from build123d import *

# Parameters (mm, degrees)
SKETCH1_W           = 260
SKETCH1_H           = 160
BOSS_EXTRUDE1_DEPTH = 10
SKETCH2_W           = 30
SKETCH2_H           = 10
BOSS_EXTRUDE2_DEPTH = 22
SKETCH3_R           = 1.5
CUT_EXTRUDE1_DEPTH  = 112
SKETCH4_W           = 30
SKETCH4_H           = 2.519449054
BOSS_EXTRUDE3_DEPTH = 10
SKETCH5_R           = 3.25
CUT_EXTRUDE4_DEPTH  = 10
SKETCH7_W           = 10
SKETCH7_H           = 10
CUT_EXTRUDE5_DEPTH  = 10
FILLET1_R           = 5
FILLET2_R           = 3


with BuildPart() as part:
    # Sketch1 → Boss-Extrude1 (new body)
    with BuildSketch(Plane(origin=(0, 0, 0), x_dir=(1, 0, 0), z_dir=(0, 1, 0))):
        Rectangle(SKETCH1_W, SKETCH1_H)
    extrude(amount=BOSS_EXTRUDE1_DEPTH)

    # Sketch2 → Boss-Extrude2 (add)
    with BuildSketch(Plane.XZ):
        with Locations((-65, 56)):
            Rectangle(SKETCH2_W, SKETCH2_H)
        with Locations((65, 56)):
            Rectangle(SKETCH2_W, SKETCH2_H)
        with Locations((65, -56)):
            Rectangle(SKETCH2_W, SKETCH2_H)
        with Locations((-65, -56)):
            Rectangle(SKETCH2_W, SKETCH2_H)
    extrude(amount=BOSS_EXTRUDE2_DEPTH)

    # Sketch3 → Cut-Extrude1 (cut)
    with BuildSketch(Plane.XY.offset(61)):
        with Locations((-65, -2.25)):
            Circle(SKETCH3_R)
        with Locations(Location((-65, -19.75, 0), (0, 0, 180))):
            Circle(SKETCH3_R)
        with Locations((65, -19.75)):
            Circle(SKETCH3_R)
        with Locations(Location((65, -2.25, 0), (0, 0, 180))):
            Circle(SKETCH3_R)
    cut_extrude1 = extrude(amount=-CUT_EXTRUDE1_DEPTH, mode=Mode.SUBTRACT)

    # Mirror1: Cut-Extrude1 across plane
    add(cut_extrude1.mirror(Plane.XY), mode=Mode.SUBTRACT)

    # Sketch4 → Boss-Extrude3 (add)
    with BuildSketch(Plane.XY.offset(61)):
        with Locations((-65, -23.259724527)):
            Rectangle(SKETCH4_W, SKETCH4_H)
        with Locations((65, -23.259724527)):
            Rectangle(SKETCH4_W, SKETCH4_H)
    boss_extrude3 = extrude(amount=-BOSS_EXTRUDE3_DEPTH)

    # Mirror3: Boss-Extrude3 across plane
    add(boss_extrude3.mirror(Plane.XY))

    # Sketch5 → Cut-Extrude4 (cut)
    with BuildSketch(Plane(origin=(0, 10, 0), x_dir=(1, 0, 0), z_dir=(0, 1, 0))):
        with Locations(Location((-36.593545043, 52.5, 0), (0, 0, 270))):
            Circle(SKETCH5_R)
        with Locations(Location((106.593545043, 52.5, 0), (0, 0, 270))):
            Circle(SKETCH5_R)
        with Locations(Location((-36.593545043, -52.5, 0), (0, 0, 270))):
            Circle(SKETCH5_R)
        with Locations(Location((106.593545043, -52.5, 0), (0, 0, 270))):
            Circle(SKETCH5_R)
    extrude(amount=-CUT_EXTRUDE4_DEPTH, mode=Mode.SUBTRACT)

    # Sketch7 → Cut-Extrude5 (cut)
    with BuildSketch(Plane(origin=(0, 10, 0), x_dir=(1, 0, 0), z_dir=(0, 1, 0))):
        with Locations((-5, 65)):
            Rectangle(SKETCH7_W, SKETCH7_H)
        with Locations((15, 65)):
            Rectangle(SKETCH7_W, SKETCH7_H)
    cut_extrude5 = extrude(amount=-CUT_EXTRUDE5_DEPTH, mode=Mode.SUBTRACT)

    # Mirror4: Cut-Extrude5 across plane
    add(cut_extrude5.mirror(Plane(origin=(0, 0, 0), x_dir=(1, 0, 0), z_dir=(0, 0, -1))), mode=Mode.SUBTRACT)

    # Fillet1
    fillet1_edges = [part.edges().sort_by_distance(p)[0] for p in [
        (130, 5, 80),
        (-130, 5, 80),
        (-130, 5, -80),
        (130, 5, -80),
    ]]
    fillet(fillet1_edges, radius=FILLET1_R)

    # Fillet2
    fillet2_edges = [part.edges().sort_by_distance(p)[0] for p in [
        (-10, 5, -60),
        (-10, 5, -70),
        (0, 5, -70),
        (0, 5, -60),
        (20, 5, -60),
        (10, 5, -60),
        (10, 5, -70),
        (20, 5, -70),
        (0, 5, 70),
        (0, 5, 60),
        (-10, 5, 60),
        (-10, 5, 70),
        (10, 5, 70),
        (20, 5, 70),
        (20, 5, 60),
        (10, 5, 60),
    ]]
    fillet(fillet2_edges, radius=FILLET2_R)


solid = part.part
Input: part model. Units: mm. Frame: model coordinates. A direction names the side the tool comes from. Give positions to 0.01 mm unless a question says otherwise; leave off trailing zeros. Order: outer loops, then holes, each group sorted by start corner. A loop starts at its lowest first (then second) coordinate and runs counter-clockwise, first axis right, second up. Notation, with made-up numbers: (-33.75, 58) - (-29.75, 58) arc R30 cw to (-29.75, 82) - close; hole circle Ø11 at (39, -33.75). An arc over 180 degrees is marked (long way). Write each question's results on one line, items separated by ' | '.
Item 1: Contact query for flat-ended pins moving along their axis: pin 1 Ø7.5 at (x, y) = (62.5, -9) entering from -Z; pin 2 Ø4 at (x, z) = (-96, 16.5) entering from -Y; pin 3 Ø7.5 at (x, y) = (63.5, -9) entering from +Z. Output: stop coordinate, or through.
A:
pin 1: stops at z = -61 | pin 2: stops at y = 0 | pin 3: stops at z = 61
Item 2: Draft query along Z for faces 5 (the cylindrical face through (105.349, 5.07, -49.498)), 6 (the cylindrical face through (-33.853, 5.07, -50.753)), 7 (the flat face through (-2, 5, 80)), 8 (the flat face through (-65, -24.519, -56)). Return one class per face: released by +Z, released by -Z, zero draft, split by the parting line, or undercut.
A:
face 5: undercut | face 6: undercut | face 7: released by +Z | face 8: zero draft
Item 3: Access query for faces 1 (the flat face through (65, -12, -51)), 2 (the flat face through (-65, -12, -61)), 3 (the flat face through (-80, -12, 56)), 4 (the flat face through (-50, -12, -56)). Directions: +Z, -Z, +X, -X, +Y, -Y. A direction counts if a zero-diameter tool reaches every point of the face in a straight line with its end or side. Return the directions, or none.
A:
face 1: +X, -X, -Y | face 2: -Z, +X, -X, -Y | face 3: +Z, -Z, -X, -Y | face 4: +Z, -Z, -Y
Item 4: Section C-C (x = 37). Return loops of the section in (y, z).
A:
outline: (0, -80) - (10, -80) - (10, 80) - (0, 80) - close
Item 5: Section A-A (y = -8.5). Return loops of the section in (x, z), and give its area (3 significant figures).
A:
outline: (-80, -61) - (-50, -61) - (-50, -51) - (-80, -51) - close; (-80, 51) - (-50, 51) - (-50, 61) - (-80, 61) - close; (50, -61) - (80, -61) - (80, -51) - (50, -51) - close; (50, 51) - (80, 51) - (80, 61) - (50, 61) - close | area: 1,200 mm^2
Item 6: Section B-B (z = 13). Return loops of the section in (x, y), and give its area (3 significant figures).
A:
outline: (-130, 0) - (130, 0) - (130, 10) - (-130, 10) - close | area: 2,600 mm^2
Item 7: Material intervals for line 1 along Y through (x, z) = (65, 56.25); line 2 along X through (y, z) = (-2, -58); line 3 along Z through (x, y) = (54, -22), sorted ascending.
A:
line 1: y = -24.52 to -21.25, -18.25 to -3.75, -0.75 to 10 | line 2: x = -80 to -66.48, -63.52 to -50, 50 to 63.52, 66.48 to 80 | line 3: z = -61 to -51, 51 to 61
